The model under review builds one solid part; all positions refer to its coordinate system, in mm. Face numbers are marked on the shaded views. A direction names the side the tool comes from. Round coordinates to 2 decimals unless told otherwise and drop trailing zeros. Order: outer loops, then holes, each group sorted by start corner. A loop starts at its lowest first (then second) coordinate and runs counter-clockwise, first axis right, second up. Notation, with made-up numbers: M 48,7.25 L 90,7.25 A25 cw 90,43.25 Z; hole C 35.25,13 d8. An arc over 180 degrees is marked long. Answer as CSV lines item,"result". Start each with the question number.
from build123d import *

# Parameters (mm, degrees)
F0_W     = 97.37
F0_H     = 114.8
F1_DEPTH = 12.7
F2_W     = 20.93
F2_H     = 38.36
F3_DEPTH = 12.701
F4_SIZE  = 2
F5_R     = 7.95
F6_DEPTH = 12.701


with BuildPart() as f1:
    # F0 (on Top) → F1 (new body)
    with BuildSketch(Plane.XY):
        Rectangle(F0_W, F0_H)
    extrude(amount=-F1_DEPTH)

    # F2 (on face) → F3 (cut, through all)
    with BuildSketch(Plane.XY):
        Rectangle(F2_W, F2_H)
    extrude(amount=-F3_DEPTH, mode=Mode.SUBTRACT)

    # F4
    f4_edges = [f1.edges().sort_by_distance(p)[0] for p in [
        (0, 19.18, -12.7),
        (10.465, 0, -12.7),
        (-10.465, 0, -12.7),
        (0, -19.18, -12.7),
    ]]
    chamfer(f4_edges, length=F4_SIZE)

    # F5 (on face) → F6 (cut, through all)
    with BuildSketch(Plane.XY):
        with Locations((0, 40)):
            Circle(F5_R)
        with Locations((30, 0)):
            Circle(F5_R)
        with Locations((-30, 0)):
            Circle(F5_R)
        with Locations((0, -40)):
            Circle(F5_R)
    extrude(amount=-F6_DEPTH, mode=Mode.SUBTRACT)


solid = f1.part
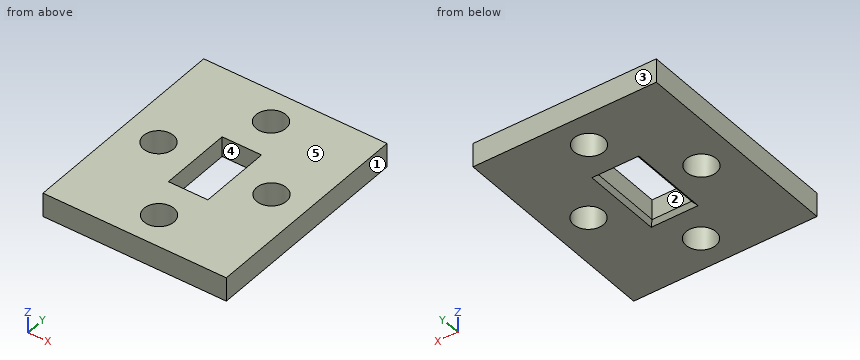
Item 1: The part is to be moulded in two halves that separate along X. For the marked faces 1, 2 and 3, say which applies: +X half, -X half, draft (parallel to the pull), parting line (faces both ways), or undercut.
Item 2: Wall thickness on probe 1 along Y at (x, z) = (0, -2.25); probe 2 along Y at (x, z) = (-4, -6.75); probe 3 along Y at (x, z) = (-30, -4.5): over which ranges is each line inside the solid? List them lowest first. Write a range as [from, to].
Item 3: Consider section B-B (y = 0). State the section outline as (x, z) points (3 decimals).
Item 4: Consider section A-A (y = -40). State the section outline as (x, z) points (3 decimals), and give its area (3 significant figures).
Item 5: Tool access review of the marked faces 4 and 5: name each direction out of +Z, -Z, +X, -X, +Y, -Y from which nothing blocks a thin tool from reaching the whole face with its end or side.
Item 6: Consider section D-D (x = -30). State the section outline as (y, z) points.
Item 7: Consider section C-C (z = -4.75). State the section outline as (x, y) points (3 decimals).
Reported:
1,face 1,"+X half"
1,face 2,"undercut"
1,face 3,"draft"
2,probe 1,"y = [-57.4, -47.95], [-32.05, -19.18], [19.18, 32.05], [47.95, 57.4]"
2,probe 2,"y = [-57.4, -46.87], [-33.13, -19.18], [19.18, 33.13], [46.87, 57.4]"
2,probe 3,"y = [-57.4, -7.95], [7.95, 57.4]"
3,outline,"M -48.685,-12.7 L -37.95,-12.7 L -37.95,0 L -48.685,0 Z; M -22.05,-12.7 L -12.465,-12.7 L -10.465,-10.7 L -10.465,0 L -22.05,0 Z; M 10.465,-10.7 L 12.465,-12.7 L 22.05,-12.7 L 22.05,0 L 10.465,0 Z; M 37.95,-12.7 L 48.685,-12.7 L 48.685,0 L 37.95,0 Z"
4,outline,"M -48.685,-12.7 L -7.95,-12.7 L -7.95,0 L -48.685,0 Z; M 7.95,-12.7 L 48.685,-12.7 L 48.685,0 L 7.95,0 Z"
4,area,"1,030 mm²"
5,face 4,"+Z, -Z"
5,face 5,"+Z, +X, -X, +Y, -Y"
6,outline,"M -57.4,-12.7 L -7.95,-12.7 L -7.95,0 L -57.4,0 Z; M 7.95,-12.7 L 57.4,-12.7 L 57.4,0 L 7.95,0 Z"
7,outline,"M -48.685,-57.4 L 48.685,-57.4 L 48.685,57.4 L -48.685,57.4 Z; hole C -30,0 d15.9; hole M -10.465,-19.18 L 10.465,-19.18 L 10.465,19.18 L -10.465,19.18 Z; hole C 0,-40 d15.9; hole C 0,40 d15.9; hole C 30,0 d15.9"
